Job drawing, mm, ordinate dimensions from the low corner. One solid piece. Round coordinates to 2 decimals unless told otherwise and drop trailing zeros. Write each loop counter-clockwise with the first axis right and the second up, starting at its lowest first coordinate (ties: lowest second). Pieces come first, ordered by that corner, then holes. Notation, with made-up numbers: M 23.5,78 L 51.5,78 A23 cw 51.5,93 Z; hole C -9,58 d1. An arc over 180 degrees is marked long. Answer as a JSON object with one key per item and string values. Group by question number.
1. Band-saw the part on B-B, the plane z = 26.5. Write the cut outline in (x, y).
2. Drill centre lines: line 1 (X direction, y = 12.7, z = 12.75); line 2 (Y direction, x = 18, z = 4.5); line 3 (X direction, y = 11.5, z = 16). Where is each one in solid material? Low to high. Write a range as from..to.
3. Drop flat-ended pins along their axis: pin 1 (3 mm diameter, centred on x = 95.25, y = 12.7, fed in from -Z); pin 2 (8 mm diameter, centred on x = 19.05, y = 12.7, fed in from -Z); pin 3 (1.7 mm diameter, centred on x = 19, z = 2, fed in from -Y). Give the stop position or say it passes through.
4. Band-saw the part on A-A, the plane x = 53. Write the cut outline in (y, z) (1 decimal), plus the area to 3 significant figures.
5. Band-saw the part on D-D, the plane x = 90.5. Write the cut outline in (y, z) (1 decimal), plus the area to 3 significant figures.
6. Band-saw the part on C-C, the plane x = 19.05. Write the cut outline in (y, z) (1 decimal), plus the area to 3 significant figures.
7. Two-plate mould, pull along Z, no slides. Class the marked faces 1, 2 and 3: +Z half, -Z half, draft (parallel to the pull), parting line (faces both ways), or undercut.
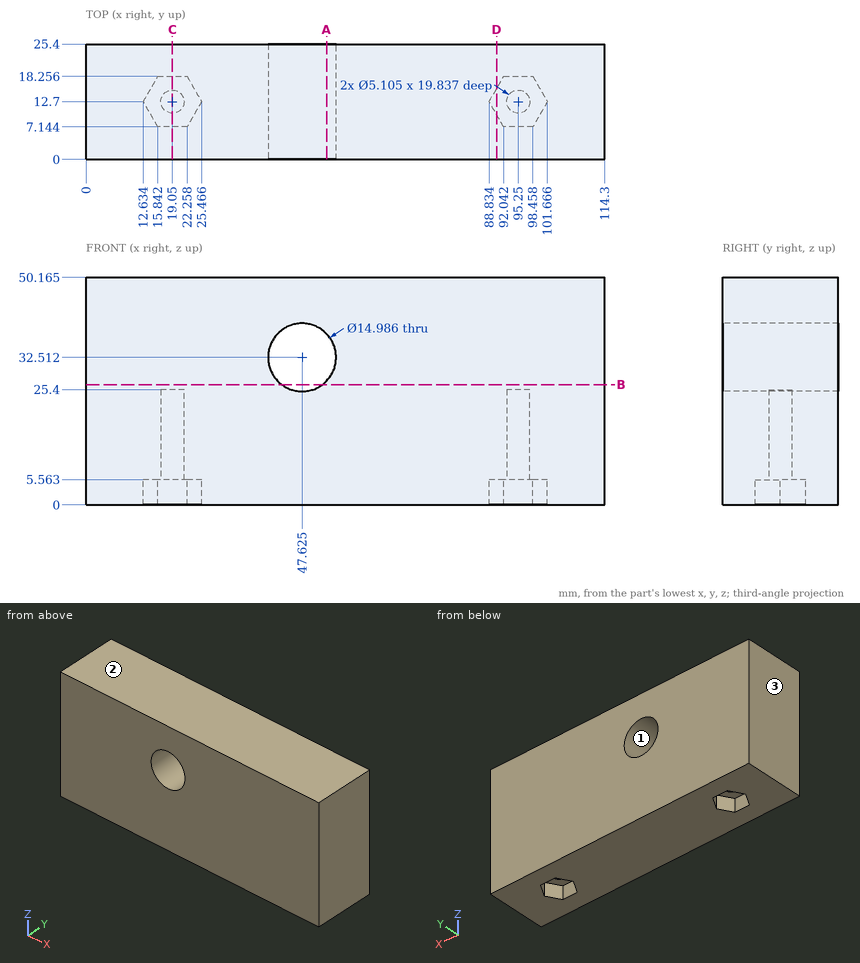
Worked answers:
{
 "1": {"outline": "M 0,0 L 43.15,0 L 43.15,25.4 L 0,25.4 Z; M 52.1,0 L 114.3,0 L 114.3,25.4 L 52.1,25.4 Z"},
 "2": {"line 1": "x = 0..16.5, 21.6..92.7, 97.8..114.3", "line 2": "y = 0..7.14, 18.26..25.4", "line 3": "x = 0..16.8, 21.3..93, 97.5..114.3"},
 "3": {"pin 1": "stops at z = 25.4", "pin 2": "stops at z = 5.56", "pin 3": "stops at y = 0"},
 "4": {"outline": "M 0,0 L 25.4,0 L 25.4,27.3 L 0,27.3 Z; M 0,37.7 L 25.4,37.7 L 25.4,50.2 L 0,50.2 Z", "area": "1,010 mm^2"},
 "5": {"outline": "M 0,0 L 9.8,0 L 9.8,5.6 L 15.6,5.6 L 15.6,0 L 25.4,0 L 25.4,50.2 L 0,50.2 Z", "area": "1,240 mm^2"},
 "6": {"outline": "M 0,0 L 7.1,0 L 7.1,5.6 L 10.1,5.6 L 10.1,25.4 L 15.3,25.4 L 15.3,5.6 L 18.3,5.6 L 18.3,0 L 25.4,0 L 25.4,50.2 L 0,50.2 Z", "area": "1,110 mm^2"},
 "7": {"face 1": "undercut", "face 2": "+Z half", "face 3": "draft"}
}
